```python
from build123d import *

# Parameters (mm, degrees)
EX_BODY_DEPTH        = 97
SK_INSERTS_M3_R      = 2
CUT_INSERTS_M3_DEPTH = 5.7
SK_VESA_M4_R         = 2.25
CUT_VESA_M4_DEPTH    = 12


with BuildPart() as part:
    # SK_Body → EX_Body (new body)
    with BuildSketch(Plane(origin=(-48.5, 0, 0), x_dir=(0, 0, -1), z_dir=(1, 0, 0))):
        Polygon((0, -19.5), (-6, -19.5), (-8.580915574, 10), (0, 10), align=None)
    extrude(amount=EX_BODY_DEPTH)

    # SK_Inserts_M3 → CUT_Inserts_M3 (cut)
    with BuildSketch(Plane.XY):
        with Locations((15, 0)):
            Circle(SK_INSERTS_M3_R)
        with Locations((-15, 0)):
            Circle(SK_INSERTS_M3_R)
    extrude(amount=CUT_INSERTS_M3_DEPTH, mode=Mode.SUBTRACT)

    # SK_VESA_M4 → CUT_VESA_M4 (cut)
    with BuildSketch(Plane.XY):
        with Locations(Location((37.5, -4.75, 0), (0, 0, 270))):
            Circle(SK_VESA_M4_R)
        with Locations(Location((-37.5, -4.75, 0), (0, 0, 270))):
            Circle(SK_VESA_M4_R)
    extrude(amount=CUT_VESA_M4_DEPTH, mode=Mode.SUBTRACT)


solid = part.part
```
The listing builds one solid part. Answer for the finished solid, in the listing's coordinates (mm). A direction names the side the tool comes from. Coordinates: 2 decimals unless noted, no trailing zeros. Loops run counter-clockwise (first coordinate to the right, second up) from the corner with the lowest first, then second, coordinate; pieces in that order, holes last. Notation, with made-up numbers: (-29.5, -29) -> (7.5, -29) arc R11 ccw to (7.5, -11) -> close; hole circle Ø9 at (-18.75, 61.25). An arc over 180 degrees is marked (long way). Return JSON: item names as keys, results as strings. Group by question number.
(1) Which of the six approach directions +Z, -Z, +X, -X, +Y, -Y give full straight-line access (tool end or side, diameter ignored) to faces 4 (the flat face through (-1, -19.5, 3)), 5 (the cylindrical face through (-16.6, -1.2, 2.8))?
(2) Determine the mould class of faces 1 (the flat face through (48.5, -5, 3)), 2 (the flat face through (15, 0, 5.7)), 3 (the flat face through (-1, 10, 4)) for opening direction Y: released by +Y, released by -Y, zero draft, split by the parting line, or undercut.
(3) A cutting plane is placed at C-C on x = -37.5. Write down the section's boundary in (y, z).
(4) A cutting plane is placed at B-B on y = -4. Write down the section's boundary in (x, z).
(5) Given pin 1 Ø3 at (x, y) = (15, 0) entering from -Z; pin 2 Ø5 at (x, y) = (17.5, 2) entering from +Z; pin 3 Ø8 at (x, y) = (-38.5, -4) entering from +Z; pin 4 Ø2.5 at (x, y) = (-37.5, -4.75) entering from -Z, each flat-ended and moving along its own axis, determine where each tip first touches the part or whether it passes through.
(6) A cutting plane is placed at D-D on x = -15. Write down the section's boundary in (y, z).
(7) A cutting plane is placed at A-A on z = 3.5. Write down the section's boundary in (x, y), and give its area (3 significant figures).
(8) Find the intervals of material crossed by probe 1 along X at (y, z) = (-4.75, 5); probe 2 along Y at (x, z) = (15, 3.8); probe 3 along Y at (x, z) = (37.5, 3.5), in increasing order. Write a range as from..to.
The answers:
{
 "1": {"face 4": "+Z, -Z, +X, -X, -Y", "face 5": "-Z"},
 "2": {"face 1": "zero draft", "face 2": "undercut", "face 3": "released by +Y"},
 "3": {"outline": "(-19.5, 0) -> (-7, 0) -> (-7, 7.09) -> (-19.5, 6) -> close; (-2.5, 0) -> (10, 0) -> (10, 8.58) -> (-2.5, 7.49) -> close"},
 "4": {"outline": "(-48.5, 0) -> (-39.62, 0) -> (-39.62, 7.36) -> (-48.5, 7.36) -> close; (-35.38, 0) -> (35.38, 0) -> (35.38, 7.36) -> (-35.38, 7.36) -> close; (39.62, 0) -> (48.5, 0) -> (48.5, 7.36) -> (39.62, 7.36) -> close"},
 "5": {"pin 1": "stops at z = 5.7", "pin 2": "stops at z = 8.1", "pin 3": "stops at z = 7.71", "pin 4": "passes through"},
 "6": {"outline": "(-19.5, 0) -> (-2, 0) -> (-2, 5.7) -> (2, 5.7) -> (2, 0) -> (10, 0) -> (10, 8.58) -> (-19.5, 6) -> close"},
 "7": {"outline": "(-48.5, -19.5) -> (48.5, -19.5) -> (48.5, 10) -> (-48.5, 10) -> close; hole circle Ø4.5 at (-37.5, -4.75); hole circle Ø4 at (-15, 0); hole circle Ø4 at (15, 0); hole circle Ø4.5 at (37.5, -4.75)", "area": "2,800 mm^2"},
 "8": {"probe 1": "x = -48.5..-39.75, -35.25..35.25, 39.75..48.5", "probe 2": "y = -19.5..-2, 2..10", "probe 3": "y = -19.5..-7, -2.5..10"}
}
